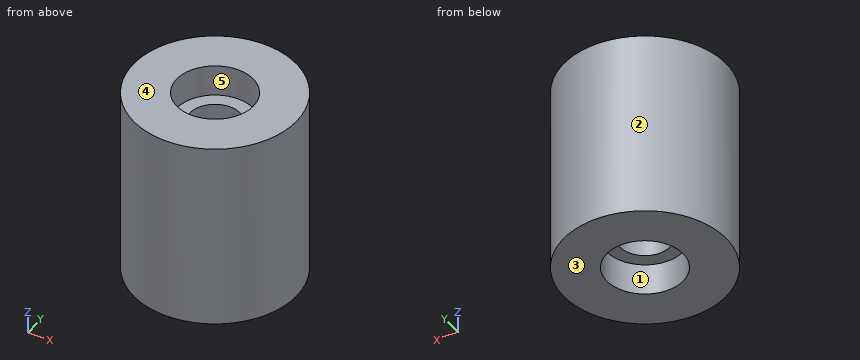
```python
from build123d import *

# Parameters (mm, degrees)
BOSS_EXTRUDE1_DEPTH      = 7.5
BOSS_EXTRUDE1_DEPTH_BACK = 7.5
SKETCH1_R                = 6.5
SKETCH1_R_2              = 2
SKETCH2_R                = 3.0625
CUT_EXTRUDE1_DEPTH       = 2.5


with BuildPart() as part:
    # Sketch1 → Boss-Extrude1 (new, two sides: drawn at the far end of the back side and taken through both)
    with BuildSketch(Plane.XY.offset(13.5).offset(-BOSS_EXTRUDE1_DEPTH_BACK)):
        with Locations((15, 0)):
            Circle(SKETCH1_R)
        with Locations((15, 0)):
            Circle(SKETCH1_R_2, mode=Mode.SUBTRACT)
    extrude(amount=BOSS_EXTRUDE1_DEPTH + BOSS_EXTRUDE1_DEPTH_BACK)

    # Sketch2 → Cut-Extrude1 (cut)
    with BuildSketch(Plane.XY.offset(21)):
        with Locations((15, 0)):
            Circle(SKETCH2_R)
    cut_extrude1 = extrude(amount=-CUT_EXTRUDE1_DEPTH, mode=Mode.SUBTRACT)

    # Mirror1: Cut-Extrude1 across plane
    add(cut_extrude1.mirror(Plane.XY.offset(13.5)), mode=Mode.SUBTRACT)


solid = part.part
```
Here's how the part is built. I have some questions about the finished solid (model axes, mm). Face numbers are marked on the shaded views. A direction names the side the tool comes from. Coordinates: 2 decimals unless noted, no trailing zeros. Order: outer loops, then holes, each group sorted by start corner. A loop starts at its lowest first (then second) coordinate and runs counter-clockwise, first axis right, second up. Notation, with made-up numbers: (3, 44.25) -> (23, 44.25) arc R13 cw to (23, 53.25) -> close; hole circle Ø6 at (17.5, -27.75). An arc over 180 degrees is marked (long way). Return JSON: item names as keys, results as strings.
1) If I drill on probe 1 along Y at (x, z) = (15, 7); probe 2 along Y at (x, z) = (13, 19); probe 3 along X at (y, z) = (-1.75, 6.75), over which ranges is the centre line in solid material (lowest first)?
Conclusion:
{"probe 1": "y = -6.5 to -3.06, 3.06 to 6.5", "probe 2": "y = -6.18 to -2.32, 2.32 to 6.18", "probe 3": "x = 8.74 to 12.49, 17.51 to 21.26"}
2) On a 3-axis mill with a long thin cutter (end or side, diameter ignored), from which of +Z, -Z, +X, -X, +Y, -Y can I reach the whole of each face in a straight line? I mean the marked faces 4 and 5. Say none if no direction works.
Conclusion:
{"face 4": "+Z, +X, -X, +Y, -Y", "face 5": "+Z"}
3) Thinking about a two-plate mould opening in Y: for the marked faces 1, 2 and 3, which applies, +Y half, -Y half, draft (parallel to the pull), parting line (faces both ways), or undercut?
Conclusion:
{"face 1": "undercut", "face 2": "parting line", "face 3": "draft"}
4) If we section it at A-A on x = 15: List the corners of the cut face in (y, z) for me, plus the area to 3 significant figures.
Conclusion:
{"outline": "(-6.5, 6) -> (-3.06, 6) -> (-3.06, 8.5) -> (-2, 8.5) -> (-2, 18.5) -> (-3.06, 18.5) -> (-3.06, 21) -> (-6.5, 21) -> close; (2, 8.5) -> (3.06, 8.5) -> (3.06, 6) -> (6.5, 6) -> (6.5, 21) -> (3.06, 21) -> (3.06, 18.5) -> (2, 18.5) -> close", "area": "124 mm²"}
5) If we section it at B-B on y = 0: List the corners of the cut face in (x, z) for me, plus the area to 3 significant figures.
Conclusion:
{"outline": "(8.5, 6) -> (11.94, 6) -> (11.94, 8.5) -> (13, 8.5) -> (13, 18.5) -> (11.94, 18.5) -> (11.94, 21) -> (8.5, 21) -> close; (17, 8.5) -> (18.06, 8.5) -> (18.06, 6) -> (21.5, 6) -> (21.5, 21) -> (18.06, 21) -> (18.06, 18.5) -> (17, 18.5) -> close", "area": "124 mm²"}
6) If we section it at C-C on z = 15: List the corners of the cut face in (x, y) for me, plus the area to 3 significant figures.
Conclusion:
{"outline": "circle Ø13 at (15, 0); hole circle Ø4 at (15, 0)", "area": "120 mm²"}
7) If we section it at D-D on y = 2.25: List the corners of the cut face in (x, z) for me.
Conclusion:
{"outline": "(8.9, 6) -> (12.92, 6) -> (12.92, 8.5) -> (17.08, 8.5) -> (17.08, 6) -> (21.1, 6) -> (21.1, 21) -> (17.08, 21) -> (17.08, 18.5) -> (12.92, 18.5) -> (12.92, 21) -> (8.9, 21) -> close"}
8) I'm going to push flat-ended pins straight in: P1, Ø5, axis at x = 15, y = 0, coming from the -Z side; P2, Ø1.8, axis at x = 15, y = -1, coming from the +Z side; P3, Ø3, axis at x = 14.5, z = 15, coming from the +Y side; P4, Ø5.5, axis at x = 15, y = 0, coming from the +Z side. Where does each tip first touch, or does it pass through?
Conclusion:
{"P1": "stops at z = 8.5", "P2": "passes through", "P3": "stops at y = 6.5", "P4": "stops at z = 18.5"}
